```python
from build123d import *

# Parameters (mm, degrees)
SKETCH1_W           = 3
SKETCH1_H           = 32
SKETCH1_H_2         = 3
SKETCH1_W_2         = 12
BOSS_EXTRUDE1_DEPTH = 15
SKETCH2_R           = 1.6
CUT_EXTRUDE1_DEPTH  = 39.392707641
SKETCH3_R           = 1.6
CUT_EXTRUDE2_DEPTH  = 40.924929555
FILLET1_R           = 3
CHAMFER1_SIZE       = 8
SKETCH6_W           = 8
SKETCH6_H           = 8
CUT_EXTRUDE5_DEPTH  = 12
FILLET2_R           = 3


with BuildPart() as part:
    # Sketch1 → Boss-Extrude1 (new body)
    with BuildSketch(Plane(origin=(0, 0, 0), x_dir=(1, 0, 0), z_dir=(0, 1, 0))):
        with Locations((1.5, 19)):
            Rectangle(SKETCH1_W, SKETCH1_H)
        with Locations((1.5, 1.5)):
            Rectangle(SKETCH1_W, SKETCH1_H_2)
        with Locations((9, 1.5)):
            Rectangle(SKETCH1_W_2, SKETCH1_H_2)
    extrude(amount=BOSS_EXTRUDE1_DEPTH)

    # Sketch2 → Cut-Extrude1 (cut, through all)
    with BuildSketch(Plane(origin=(0, 0, -3), x_dir=(-1, 0, 0), z_dir=(0, 0, -1))):
        with Locations((-9, 7.5)):
            Circle(SKETCH2_R)
    extrude(amount=-CUT_EXTRUDE1_DEPTH, mode=Mode.SUBTRACT)

    # Sketch3 → Cut-Extrude2 (cut, through all)
    with BuildSketch(Plane(origin=(3, 0, 0), x_dir=(0, 0, -1), z_dir=(1, 0, 0))):
        with Locations((13, 7.5)):
            Circle(SKETCH3_R)
        with Locations((29, 7.5)):
            Circle(SKETCH3_R)
    extrude(amount=-CUT_EXTRUDE2_DEPTH, mode=Mode.SUBTRACT)

    # Fillet1
    fillet1_edges = [part.edges().sort_by_distance(p)[0] for p in [
        (15, 15, -1.5),
        (1.5, 15, -35),
        (1.5, 0, -35),
        (15, 0, -1.5),
    ]]
    fillet(fillet1_edges, radius=FILLET1_R)

    # Chamfer1
    # the kernel refuses this chamfer: 8 mm, written as the material it adds along each edge
    with BuildSketch(Plane(origin=(3, 0, -3), x_dir=(-0.027495876610586382, 0, -0.9996219169112968), z_dir=(0, 1, 0))) as chamfer1_piece_1_section:
        Polygon((CHAMFER1_SIZE * 0.999621916911, -CHAMFER1_SIZE * 0.0274958766106), (-CHAMFER1_SIZE * 0.0274958766106, -CHAMFER1_SIZE * 0.999621916911), (0, 0), align=None)
    chamfer1_piece_1 = extrude(amount=15, mode=Mode.PRIVATE)
    chamfer1_piece_1 = chamfer1_piece_1 - Plane(origin=(9, 7.5, -5.695402836), x_dir=(-1, 0, 0), z_dir=(0, 0, -1)) * Cylinder(1.6, 62, mode=Mode.PRIVATE)
    add(chamfer1_piece_1)

    # Sketch6 → Cut-Extrude5 (cut)
    with BuildSketch(Plane(origin=(15, 0, 0), x_dir=(0, 0, -1), z_dir=(1, 0, 0))):
        with Locations((7, 7.5)):
            Rectangle(SKETCH6_W, SKETCH6_H)
    extrude(amount=-CUT_EXTRUDE5_DEPTH, mode=Mode.SUBTRACT)

    # Fillet2
    fillet2_edges = [part.edges().sort_by_distance(p)[0] for p in [
        (3, 7.5, -3),
        (11, 1.75, -3),
        (3, 1.75, -11),
        (3, 13.25, -11),
        (11, 13.25, -3),
    ]]
    fillet(fillet2_edges, radius=FILLET2_R)


solid = part.part
```
CAD build for the part. Positions are in the model's coordinates, mm. A direction names the side the tool comes from. Round coordinates to 2 decimals unless told otherwise and drop trailing zeros. Order: outer loops, then holes, each group sorted by start corner. A loop starts at its lowest first (then second) coordinate and runs counter-clockwise, first axis right, second up. Notation, with made-up numbers: (89.5, 67) - (119.5, 67) arc R14 ccw to (119.5, 89) - close; hole circle Ø1 at (16.5, 3.25). An arc over 180 degrees is marked (long way). Answer as CSV lines item,"result". Start each with the question number.
1. Saw through at B-B, the plane z = -29. Write the cut outline in (x, y).
2. Saw through at A-A, the plane y = 7.5. Write the cut outline in (x, z), and give its area (3 significant figures).
3. Saw through at D-D, the plane x = 1.5. Write the cut outline in (y, z).
4. Pin check, flat tips, straight feed: pin 1 (3 mm diameter, centred on y = 7.5, z = -13, fed in from -X); pin 2 (6 mm diameter, centred on y = 2, z = -15.5, fed in from +X); pin 3 (8 mm diameter, centred on y = 11, z = -9, fed in from +X). Stop position of each tip, or through.
5. Tool access for faces 1 (the face through (7, 2, -7)), 2 (the face through (3.86, 7.56, -3.9)): list every direction of +Z, -Z, +X, -X, +Y, -Y with a clear straight run to the whole face (end or side of a thin tool).
6. Saw through at C-C, the plane x = 9. Write the cut outline in (y, z).
7. Pull direction Z, two halves, no side cores. Call faces 3 (the face through (6, 3.5, -6)), 4 (the face through (3.235, 1.774, -11.079)), 5 (the face through (1.52, 6.53, -27.73)): +Z half, -Z half, draft (parallel to the pull), parting line (faces both ways), or undercut.
8. Drill centre lines: L1, parallel to Z at x = 1.5, y = 8; L2, parallel to Y at x = 2, z = -29; L3, parallel to Z at x = 13.25, y = 9.75. Where is each one in solid material? Low to high. Write a range as [from, to].
Model answer:
1,outline,"(0, 0) - (3, 0) - (3, 5.9) - (0, 5.9) - close; (0, 9.1) - (3, 9.1) - (3, 15) - (0, 15) - close"
2,outline,"(0, -35) - (3, -35) - (3, -30.6) - (0, -30.6) - close; (0, -27.4) - (3, -27.4) - (3, -14.6) - (0, -14.6) - close; (0, -11.4) - (3, -11.4) - (3, -6) arc R3 cw to (6, -3) - (7.4, -3) - (7.4, 0) - (0, 0) - close; (10.6, -3) - (15, -3) - (15, 0) - (10.6, 0) - close"
2,area,"114 mm²"
3,outline,"(0, -32) arc R3 ccw to (3, -35) - (12, -35) arc R3 ccw to (15, -32) - (15, 0) - (0, 0) - close; hole circle Ø3.2 at (7.5, -29); hole circle Ø3.2 at (7.5, -13)"
4,pin 1,"passes through"
4,pin 2,"stops at x = 3"
4,pin 3,"stops at x = 8.97"
5,face 1,"-Z, +X, +Y, -Y"
5,face 2,"-Z, +X"
6,outline,"(0, -5) - (3.5, -5) - (3.5, -3) - (5.9, -3) - (5.9, 0) - (0, 0) - close; (9.1, -3) - (11.5, -3) - (11.5, -5) - (15, -5) - (15, 0) - (9.1, 0) - close"
7,face 3,"draft"
7,face 4,"-Z half"
7,face 5,"undercut"
8,L1,"z = [-35, -30.52], [-27.48, -14.52], [-11.48, 0]"
8,L2,"y = [0, 5.9], [9.1, 15]"
8,L3,"z = [-3, 0]"
